The listing builds one solid part. Answer for the finished solid, in the listing's coordinates (mm). Give positions to 0.01 mm unless a question says otherwise; leave off trailing zeros. Order: outer loops, then holes, each group sorted by start corner. A loop starts at its lowest first (then second) coordinate and runs counter-clockwise, first axis right, second up. Notation, with made-up numbers: (-27, 37) - (-3, 37) arc R16 ccw to (-3, 65) - close; hole circle Ø1 at (48.5, 18). An arc over 180 degrees is marked (long way). Use a Markdown table: item, result. Add a question column.
1) Find section C-C, the plane x = 4.5. Determine the outline of the cut face in (y, z).
2) Find section D-D, the plane y = 65.5. Determine the outline of the cut face in (x, z), plus the area to 3 significant figures.
3) Find section A-A, the plane z = -1.5. Determine the outline of the cut face in (x, y).
4) Find section B-B, the plane y = 26.5. Determine the outline of the cut face in (x, z).
5) Straight lines are drawn through the part: line 1 (Y direction, x = 0, z = -4.7); line 2 (Z direction, x = 1, y = 5); line 3 (X direction, y = -59, z = -1.5). For each, find the intervals that lie inside material, in ascending order.
6) A flat-ended cylindrical pin translates along its axis: pin 1 (1.5 mm diameter, centred on x = 3, z = 2.5, fed in from -Y). Find the tip coordinate at first contact, or state that the pin passes through.
from build123d import *

# Parameters (mm, degrees)
SKETCH_1_W          = 15
SKETCH_1_H          = 10
SKETCH_1_W_2        = 12.6
SKETCH_1_H_2        = 7.6
EXTRUDE_1_DEPTH     = 70.5
SKETCH_2_R          = 1.6
CUT_EXTRUDE_1_DEPTH = 100


with BuildPart() as part:
    # ｽｹｯﾁ1 → ﾎﾞｽ - 押し出し1 (new, symmetric)
    with BuildSketch(Plane(origin=(0, 0, 0), x_dir=(1, 0, 0), z_dir=(0, 1, 0))):
        Rectangle(SKETCH_1_W, SKETCH_1_H)
        Rectangle(SKETCH_1_W_2, SKETCH_1_H_2, mode=Mode.SUBTRACT)
    extrude(amount=EXTRUDE_1_DEPTH, both=True)

    # ｽｹｯﾁ2 → ｶｯﾄ - 押し出し1 (cut)
    with BuildSketch(Plane(origin=(0, 0, -5), x_dir=(-1, 0, 0), z_dir=(0, 0, -1))):
        with Locations((0, -65.5)):
            Circle(SKETCH_2_R)
        with Locations((0, -45.5)):
            Circle(SKETCH_2_R)
        with Locations(Location((0, 45.5, 0), (0, 0, 180))):
            Circle(SKETCH_2_R)
        with Locations(Location((0, 65.5, 0), (0, 0, 180))):
            Circle(SKETCH_2_R)
    extrude(amount=-CUT_EXTRUDE_1_DEPTH, mode=Mode.SUBTRACT)


solid = part.part
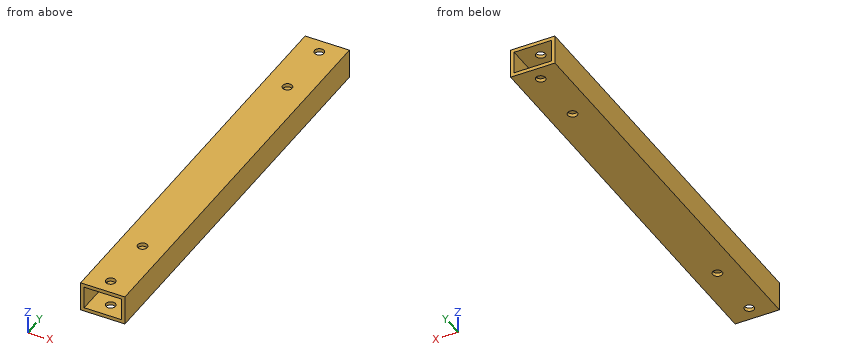
The answers:
| question | item | result |
|---|---|---|
| 1 | outline | (-70.5, -5) - (70.5, -5) - (70.5, -3.8) - (-70.5, -3.8) - close; (-70.5, 3.8) - (70.5, 3.8) - (70.5, 5) - (-70.5, 5) - close |
| 2 | outline | (-7.5, -5) - (-1.6, -5) - (-1.6, -3.8) - (-6.3, -3.8) - (-6.3, 3.8) - (-1.6, 3.8) - (-1.6, 5) - (-7.5, 5) - close; (1.6, -5) - (7.5, -5) - (7.5, 5) - (1.6, 5) - (1.6, 3.8) - (6.3, 3.8) - (6.3, -3.8) - (1.6, -3.8) - close |
| 2 | area | 46.6 mm2 |
| 3 | outline | (-7.5, -70.5) - (-6.3, -70.5) - (-6.3, 70.5) - (-7.5, 70.5) - close; (6.3, -70.5) - (7.5, -70.5) - (7.5, 70.5) - (6.3, 70.5) - close |
| 4 | outline | (-7.5, -5) - (7.5, -5) - (7.5, 5) - (-7.5, 5) - close; hole (-6.3, -3.8) - (6.3, -3.8) - (6.3, 3.8) - (-6.3, 3.8) - close |
| 5 | line 1 | -70.5 to -67.1, -63.9 to -47.1, -43.9 to 43.9, 47.1 to 63.9, 67.1 to 70.5 |
| 5 | line 2 | -5 to -3.8, 3.8 to 5 |
| 5 | line 3 | -7.5 to -6.3, 6.3 to 7.5 |
| 6 | pin 1 | through |
